```python
from build123d import *

# Parameters (mm, degrees)
SKETCH1_R                 = 4.7625
BOSS_EXTRUDE1_DEPTH       = 1.5875
M4_CLEARANCE_HOLE1_D      = 4.3
M3X0_5_TAPPED_HOLE1_D     = 2.5
M3X0_5_TAPPED_HOLE1_DEPTH = 3.175
FILLET1_R                 = 6.35


with BuildPart() as part:
    # Sketch1 → Boss-Extrude1 (new, symmetric)
    with BuildSketch(Plane(origin=(0, 0, 0), x_dir=(1, 0, 0), z_dir=(0, 1, 0))):
        with BuildLine():
            Line((-8.635805476, -12.264699906), (8.978028762, -24.666931296))
            ThreePointArc((8.978028762, -24.666931296), (26.25, 0), (8.978028762, 24.666931296))
            Line((8.978028762, 24.666931296), (-8.635805476, 12.264699906))
            ThreePointArc((-8.635805476, 12.264699906), (-15, 0), (-8.635805476, -12.264699906))
        make_face()
        with Locations(Location((0, 0, 0), (0, 0, 270))):
            Circle(SKETCH1_R, mode=Mode.SUBTRACT)
    extrude(amount=BOSS_EXTRUDE1_DEPTH, both=True)

    # M4 Clearance Hole1 (through all)
    with Locations(Plane(origin=(0, 1.5875, 0), x_dir=(1, 0, 0), z_dir=(0, 1, 0))):
        with Locations((10.75, -18.619546181), (10.75, 18.619546181)):
            Hole(M4_CLEARANCE_HOLE1_D / 2)

    # M3x0.5 Tapped Hole1
    with Locations(Plane(origin=(0, 1.5875, 0), x_dir=(1, 0, 0), z_dir=(0, 1, 0))):
        with Locations((0, 0), (15.75, -10.48), (15.75, 10.48)):
            Hole(M3X0_5_TAPPED_HOLE1_D / 2, depth=M3X0_5_TAPPED_HOLE1_DEPTH)

    # Fillet1
    fillet1_edges = [part.edges().sort_by_distance(p)[0] for p in [
        (8.978028762, 0, -24.666931296),
        (8.978028762, 0, 24.666931296),
    ]]
    fillet(fillet1_edges, radius=FILLET1_R)


solid = part.part
```
Model file for the job. Use its own axes, mm. Coordinates: 2 decimals unless noted, no trailing zeros. Write each loop counter-clockwise with the first axis right and the second up, starting at its lowest first coordinate (ties: lowest second). Pieces come first, ordered by that corner, then holes. Notation, with made-up numbers: (3, 41.25) - (51, 41.25) arc R4 ccw to (51, 46.25) - close; hole circle Ø5 at (18, 2). An arc over 180 degrees is marked (long way). One line per question, with ' | ' between items. Start each with the question number.
Q1. Cut at C-C, the plane y = 0.5. Give the number of separate pieces and of enclosed holes in the cut face, then the cut area to 3 significant figures.
Q2. Cut at B-B, the plane x = 16. List the corners of the cut face in (y, z).
Q3. Cut at A-A, the plane z = 0. List the corners of the cut face in (x, y).
Q4. Pin check, flat tip, straight feed: pin 1 (1.5 mm diameter, centred on x = -10, y = -1.5, fed in from -Z). Stop position of the tip, or through.
Q5. Drill centre lines: line 1 (Z direction, x = 10.75, y = -0.25); line 2 (Z direction, x = 15.75, y = -0.55); line 3 (X direction, y = -0.4, z = 0). Where is each one in solid material? Low to high. Write a range as [from, to].
Q6. Cut at D-D, the plane z = -11. List the corners of the cut face in (x, y).
Q7. Pull direction X, two halves, no side cores. Call faces 1 (the face through (9.76, -0.02, 20.53)), 2 (the face through (-1.412, 0.022, 17.351)), 3 (the face through (26.247, 0.022, 0.391)), 4 (the face through (9.388, 0.022, -23.734)): pulls with the +X half, pulls with the -X half, needs draft (parallel to the pull), parting line crosses it, or undercut.
Answer below:
1) separate pieces: 1 | enclosed holes: 5 | area: 1,270 mm^2
2) outline: (-1.59, -20.81) - (1.59, -20.81) - (1.59, -11.7) - (-1.59, -11.7) - close; (-1.59, -9.26) - (1.59, -9.26) - (1.59, 9.26) - (-1.59, 9.26) - close; (-1.59, 11.7) - (1.59, 11.7) - (1.59, 20.81) - (-1.59, 20.81) - close
3) outline: (-15, -1.59) - (-4.76, -1.59) - (-4.76, 1.59) - (-15, 1.59) - close; (4.76, -1.59) - (26.25, -1.59) - (26.25, 1.59) - (4.76, 1.59) - close
4) pin 1: z = -11.81
5) line 1: [-23.65, -20.77], [-16.47, 16.47], [20.77, 23.65] | line 2: [-21, -11.73], [-9.23, 9.23], [11.73, 21] | line 3: [-15, -4.76], [4.76, 26.25]
6) outline: (-10.2, -1.59) - (14.61, -1.59) - (14.61, 1.59) - (-10.2, 1.59) - close; (16.89, -1.59) - (23.83, -1.59) - (23.83, 1.59) - (16.89, 1.59) - close
7) face 1: undercut | face 2: pulls with the -X half | face 3: pulls with the +X half | face 4: parting line crosses it
